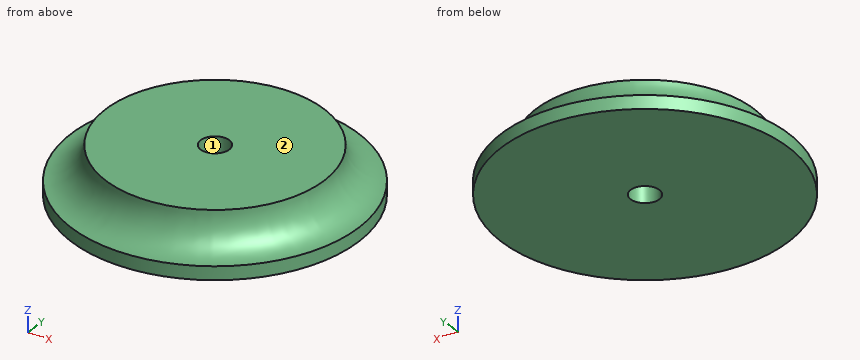
from build123d import *

# Parameters (mm, degrees)
SKETCH9_R                  = 38.1
BOSS_EXTRUDE2_DEPTH        = 3.556
BOSS_EXTRUDE3_START        = 3.556
SKETCH10_R                 = 38.1
BOSS_EXTRUDE3_DEPTH        = 3.556
F_3_4_0_3_DIAMETER_HOLE1_D = 7.62
CUT_EXTRUDE1_DEPTH         = 59.141038312
CUT_EXTRUDE1_DEPTH_BACK    = 59.141038312
SKETCH16_W                 = 76.2
SKETCH16_H                 = 12.7


with BuildPart() as part:
    # Sketch5 → Revolve1 (revolve)
    with BuildSketch(Plane(origin=(0, 0, 0), x_dir=(1, 0, 0), z_dir=(0, 1, 0)), mode=Mode.PRIVATE) as revolve1_sk:
        with BuildLine():
            Line((0, 0), (-38.1, 0))
            ThreePointArc((-38.1, 0), (-28.956, 9.144), (-38.1, 18.288))
            Line((-38.1, 18.288), (0, 18.288))
            Line((0, 18.288), (0, 0))
        make_face()
    revolve(revolve1_sk.sketch.rotate(Axis((0, 0, 0), (0, 0, -1)), 180), axis=Axis((0, 0, 0), (0, 0, -1)))

    # Sketch9 → Boss-Extrude2 (add)
    with BuildSketch(Plane.XY):
        Circle(SKETCH9_R)
    extrude(amount=BOSS_EXTRUDE2_DEPTH)

    # Sketch10 → Boss-Extrude3 (add)
    with BuildSketch(Plane(origin=(0, 0, -18.288), x_dir=(-1, 0, 0), z_dir=(0, 0, -1)).offset(BOSS_EXTRUDE3_START)):
        with Locations(Location((0, 0, 0), (0, 0, 180))):
            Circle(SKETCH10_R)
    extrude(amount=-BOSS_EXTRUDE3_DEPTH)

    # 3/4 (0.3) Diameter Hole1 (through all)
    with Locations(Plane.XY.offset(3.556)):
        with Locations((0, 0)):
            Hole(F_3_4_0_3_DIAMETER_HOLE1_D / 2)

    # Sketch16 → Cut-Extrude1 (cut, two sides: drawn at the far end of the back side and taken through both)
    with BuildSketch(Plane(origin=(0, 0, 0), x_dir=(1, 0, 0), z_dir=(0, 1, 0)).offset(-CUT_EXTRUDE1_DEPTH_BACK)):
        with Locations((0, 2.794)):
            Rectangle(SKETCH16_W, SKETCH16_H)
    extrude(amount=CUT_EXTRUDE1_DEPTH + CUT_EXTRUDE1_DEPTH_BACK, mode=Mode.SUBTRACT)


solid = part.part
Geometry check sheet. Reference: the model listing, model coordinates, mm. Face numbers are marked on the shaded views. Round coordinates to 2 decimals unless told otherwise and drop trailing zeros. Write each loop counter-clockwise with the first axis right and the second up, starting at its lowest first coordinate (ties: lowest second). Pieces come first, ordered by that corner, then holes. Notation, with made-up numbers: (13.5, 81.5) - (45.5, 81.5) arc R13 cw to (45.5, 96.5) - close; hole circle Ø3 at (16.25, -27.75). An arc over 180 degrees is marked (long way). One line per item, written item: value.
1. Mould release check, pull along X, two halves, no side actions. Record for the marked faces 1 and 2: released by +X, released by -X, zero draft, split by the parting line, or undercut.
The answers:
face 1: undercut
face 2: zero draft
2. Depth check by flat-ended pin: pin 1 Ø6 at (x, z) = (-7.5, -18.5) entering from +Y; pin 2 Ø1.5 at (y, z) = (21, -19) entering from +X; pin 3 Ø1.5 at (x, z) = (-29, -20) entering from +Y. Enter the tip coordinate at first touch or a pass-through.
The answers:
pin 1: stops at y = 37.83
pin 2: stops at x = 32.27
pin 3: stops at y = 25.56
3. Cross-section at A-A on y = 0. Record the boundary of the cut face in (x, z).
The answers:
outline: (-38.1, -21.84) - (-3.81, -21.84) - (-3.81, -9.14) - (-28.96, -9.14) arc R9.14 cw to (-38.1, -18.29) - close; (3.81, -21.84) - (38.1, -21.84) - (38.1, -18.29) arc R9.14 cw to (28.96, -9.14) - (3.81, -9.14) - close
4. Cross-section at C-C on z = -20.25. Record the boundary of the cut face in (x, y), and give its area (3 significant figures).
The answers:
outline: circle Ø76.2 at (0, 0); hole circle Ø7.62 at (0, 0)
area: 4,510 mm^2
5. Scan lines: L1, parallel to Z at x = 35, y = 14; L2, parallel to Y at x = 0, z = -13; L3, parallel to X at y = -3, z = -16.75. Record each from-to range of solid material in increasing order.
The answers:
L1: z = -21.84 to -18.28
L2: y = -29.81 to -3.81, 3.81 to 29.81
L3: x = -32.89 to -2.35, 2.35 to 32.89
6. Cross-section at D-D on z = -16. Record the boundary of the cut face in (x, y).
The answers:
outline: circle Ø64.1 at (0, 0); hole circle Ø7.62 at (0, 0)
